```python
from build123d import *

# Parameters (mm, degrees)
SKETCH1_R                  = 95.25
BOSS_EXTRUDE1_DEPTH        = 4.7625
F_12_24_TAPPED_HOLE1_D     = 4.4958
F_12_24_TAPPED_HOLE1_DEPTH = 14.224


with BuildPart() as part:
    # Sketch1 → Boss-Extrude1 (new body)
    with BuildSketch(Plane.XY):
        Circle(SKETCH1_R)
    extrude(amount=BOSS_EXTRUDE1_DEPTH)

    # #12-24 Tapped Hole1
    with Locations(Plane.XY.offset(4.7625)):
        with Locations((0, 79.375), (-79.375, 0), (79.375, 0), (0, -79.375)):
            Hole(F_12_24_TAPPED_HOLE1_D / 2, depth=F_12_24_TAPPED_HOLE1_DEPTH)


solid = part.part
```
The listing builds one solid part. Answer for the finished solid, in the listing's coordinates (mm). Coordinates: 2 decimals unless noted, no trailing zeros. Write each loop counter-clockwise with the first axis right and the second up, starting at its lowest first coordinate (ties: lowest second). Pieces come first, ordered by that corner, then holes. Notation, with made-up numbers: (4, 87.5) -> (15, 87.5) arc R26 cw to (15, 109.5) -> close; hole circle Ø1 at (71.5, -30). An arc over 180 degrees is marked (long way). Write each question's results on one line, items separated by ' | '. Start each with the question number.
1) Flat-ended cylindrical pins translate along their axes: pin 1 Ø1.5 at (y, z) = (65, 2.5) entering from +X; pin 2 Ø4 at (x, y) = (-79.375, 0) entering from -Z; pin 3 Ø2 at (y, z) = (13.5, 1) entering from -X; pin 4 Ø7 at (x, y) = (0, -79.375) entering from -Z. Find the tip coordinate at first contact, or state that the pin passes through.
2) Straight lines are drawn through the part: probe 1 along Y at (x, z) = (0, 3.45); probe 2 along X at (y, z) = (78, 0.85); probe 3 along Y at (x, z) = (-19, 2.75). For each, find the intervals that lie inside material, in ascending order.
3) For a pull along Y with two mould halves and no side action, classify faces 1 (the cylindrical face through (-75.587, -57.958, 2.348)), 2 (the flat face through (-1, 1, 0)), 3 (the cylindrical face through (1.784, -80.743, 2.348)), 4 (the cylindrical face through (-77.13, 0.1, 2.35)) as +Y half, -Y half, draft (parallel to the pull), parting line (faces both ways), or undercut.
4) A cutting plane is placed at C-C (z = 2.5). Determine the outline of the cut face in (x, y) (3 decimals).
5) A cutting plane is placed at D-D (x = -34). Determine the outline of the cut face in (y, z).
6) A cutting plane is placed at A-A (x = 0). Determine the outline of the cut face in (y, z), then the cut area to 3 significant figures.
Values follow:
1) pin 1: x = 70.32 | pin 2: through | pin 3: x = -94.43 | pin 4: z = 0
2) probe 1: -95.25 to -81.62, -77.13 to 77.13, 81.62 to 95.25 | probe 2: -54.67 to -1.78, 1.78 to 54.67 | probe 3: -93.34 to 93.34
3) face 1: parting line | face 2: draft | face 3: undercut | face 4: undercut
4) outline: circle Ø190.5 at (0, 0); hole circle Ø4.496 at (-79.375, 0); hole circle Ø4.496 at (0, -79.375); hole circle Ø4.496 at (0, 79.375); hole circle Ø4.496 at (79.375, 0)
5) outline: (-88.98, 0) -> (88.98, 0) -> (88.98, 4.76) -> (-88.98, 4.76) -> close
6) outline: (-95.25, 0) -> (-81.62, 0) -> (-81.62, 4.76) -> (-95.25, 4.76) -> close; (-77.13, 0) -> (77.13, 0) -> (77.13, 4.76) -> (-77.13, 4.76) -> close; (81.62, 0) -> (95.25, 0) -> (95.25, 4.76) -> (81.62, 4.76) -> close | area: 864 mm²
